Design review of the part built by this model. Coordinates are the model's own, in mm. A direction names the side the tool comes from. Round coordinates to 2 decimals unless told otherwise and drop trailing zeros. Loops run counter-clockwise (first coordinate to the right, second up) from the corner with the lowest first, then second, coordinate; pieces in that order, holes last. Notation, with made-up numbers: (40.25, 57.5) -> (86.25, 57.5) arc R17 cw to (86.25, 68.5) -> close; hole circle Ø8 at (36.5, 80.25). An arc over 180 degrees is marked (long way). Use a Markdown table: item, result. Add a question column.
from build123d import *

# Parameters (mm, degrees)
CYLINDER267_R                = 2
CYLINDER267_DEPTH            = 10
CYLINDER267_PITCH_ANGLE      = 90
BOX001027045199_W            = 3
BOX001027045199_H            = 8
BOX001027045199_DEPTH        = 8
FILLET045_R                  = 3
CUT239_PITCH_ANGLE           = 90
CYLINDER103_R                = 1.4
CYLINDER103_DEPTH            = 19
CYLINDER103_ROLL_ANGLE       = 90
CYLINDER105_R                = 1.4
CYLINDER105_DEPTH            = 19
CYLINDER105_ROLL_ANGLE       = 90
CYLINDER106_R                = 1.4
CYLINDER106_DEPTH            = 19
CYLINDER106_ROLL_ANGLE       = 90
CYLINDER027_R                = 1.4
CYLINDER027_DEPTH            = 19
CYLINDER027_ROLL_ANGLE       = 90
CYLINDER098_R                = 1
CYLINDER098_DEPTH            = 30
CYLINDER099_R                = 1
CYLINDER099_DEPTH            = 30
BOX001007_W                  = 4
BOX001007_H                  = 4.2
BOX001007_DEPTH              = 27
CYLINDER097_R                = 2.1
CYLINDER097_DEPTH            = 30
CYLINDER023_R                = 2.1
CYLINDER023_DEPTH            = 30
CYLINDER100_R                = 1
CYLINDER100_DEPTH            = 30
BOX001008_W                  = 4
BOX001008_H                  = 2
BOX001008_DEPTH              = 27
CYLINDER101_R                = 1
CYLINDER101_DEPTH            = 30
BOX001009_W                  = 4
BOX001009_H                  = 2
BOX001009_DEPTH              = 27
CYLINDER093_R                = 3.5
CYLINDER093_DEPTH            = 30
CYLINDER094_R                = 4.7
CYLINDER094_DEPTH            = 30
CYLINDER095_R                = 10
CYLINDER095_DEPTH            = 30
CYLINDER102_R                = 10
CYLINDER102_DEPTH            = 30
CYLINDER096_R                = 10
CYLINDER096_DEPTH            = 30
BOX001006_W                  = 39
BOX001006_H                  = 24
BOX001006_DEPTH              = 10
CHAMFER008_SIZE              = 1
CHAMFER014_SIZE              = 0.5
FUSION112154_ROLL_ANGLE      = 180
FUSION112154_PLACEMENT_ANGLE = -90


with BuildPart() as cylinder285:
    # Cylinder267 → Cylinder267 (new body)
    with BuildSketch(Plane.XY):
        Circle(CYLINDER267_R)
    extrude(amount=CYLINDER267_DEPTH)


with BuildPart() as cylinder285_1:
    # Cylinder267 pitch: moved
    add(cylinder285.part.rotate(Axis((0, 0, 0), (0, 1, 0)), CYLINDER267_PITCH_ANGLE))


with BuildPart() as cylinder285_2:
    # Cylinder267 placement: moved
    add(cylinder285_1.part.moved(Location((-3, 4, 4.5))))


with BuildPart() as cut239:
    # Box001027045199 → Box001027045199 (new body)
    with BuildSketch(Plane.XY):
        with Locations((1.5, 4)):
            Rectangle(BOX001027045199_W, BOX001027045199_H)
    extrude(amount=BOX001027045199_DEPTH)

    # Fillet045
    fillet045_edges = [cut239.edges().sort_by_distance(p)[0] for p in [
        (1.5, 0, 8),
        (1.5, 8, 8),
    ]]
    fillet(fillet045_edges, radius=FILLET045_R)

    # Cut239: cut Cylinder285
    add(cylinder285_2.part, mode=Mode.SUBTRACT)


with BuildPart() as cut239_1:
    # Cut239 pitch: moved
    add(cut239.part.rotate(Axis((0, 0, 0), (0, 1, 0)), CUT239_PITCH_ANGLE))


with BuildPart() as cut239_2:
    # Cut239 placement: moved
    add(cut239_1.part.moved(Location((25, -4, 10))))


with BuildPart() as cylinder103:
    # Cylinder103 → Cylinder103 (new body)
    with BuildSketch(Plane.XY):
        Circle(CYLINDER103_R)
    extrude(amount=CYLINDER103_DEPTH)


with BuildPart() as cylinder103_1:
    # Cylinder103 roll: moved
    add(cylinder103.part.rotate(Axis((0, 0, 0), (1, 0, 0)), CYLINDER103_ROLL_ANGLE))


with BuildPart() as cylinder103_2:
    # Cylinder103 placement: moved
    add(cylinder103_1.part.moved(Location((4, 24, 6))))


with BuildPart() as cylinder105:
    # Cylinder105 → Cylinder105 (new body)
    with BuildSketch(Plane.XY):
        Circle(CYLINDER105_R)
    extrude(amount=CYLINDER105_DEPTH)


with BuildPart() as cylinder105_1:
    # Cylinder105 roll: moved
    add(cylinder105.part.rotate(Axis((0, 0, 0), (1, 0, 0)), CYLINDER105_ROLL_ANGLE))


with BuildPart() as cylinder105_2:
    # Cylinder105 placement: moved
    add(cylinder105_1.part.moved(Location((-4, 24, 6))))


with BuildPart() as part_mirroring011:
    # Part__Mirroring011: instance of Cylinder105
    add(cylinder105_2.part.mirror(Plane(origin=(0, 0, 0), x_dir=(1, 0, 0), z_dir=(0, 1, 0))))


with BuildPart() as cylinder106:
    # Cylinder106 → Cylinder106 (new body)
    with BuildSketch(Plane.XY):
        Circle(CYLINDER106_R)
    extrude(amount=CYLINDER106_DEPTH)


with BuildPart() as cylinder106_1:
    # Cylinder106 roll: moved
    add(cylinder106.part.rotate(Axis((0, 0, 0), (1, 0, 0)), CYLINDER106_ROLL_ANGLE))


with BuildPart() as cylinder106_2:
    # Cylinder106 placement: moved
    add(cylinder106_1.part.moved(Location((4, 24, 6))))


with BuildPart() as part_mirroring012:
    # Part__Mirroring012: instance of Cylinder106
    add(cylinder106_2.part.mirror(Plane(origin=(0, 0, 0), x_dir=(1, 0, 0), z_dir=(0, 1, 0))))


with BuildPart() as m3_tap_a:
    # Cylinder027 → Cylinder027 (new body)
    with BuildSketch(Plane.XY):
        Circle(CYLINDER027_R)
    extrude(amount=CYLINDER027_DEPTH)


with BuildPart() as m3_tap_a_1:
    # Cylinder027 roll: moved
    add(m3_tap_a.part.rotate(Axis((0, 0, 0), (1, 0, 0)), CYLINDER027_ROLL_ANGLE))


with BuildPart() as m3_tap_a_2:
    # Cylinder027 placement: moved
    add(m3_tap_a_1.part.moved(Location((-4, 24, 6))))

    # Fusion062: union Cylinder103, Part__Mirroring011, Part__Mirroring012
    add(cylinder103_2.part)
    add(part_mirroring011.part)
    add(part_mirroring012.part)


with BuildPart() as cylinder109:
    # Cylinder098 → Cylinder098 (new body)
    with BuildSketch(Plane(origin=(17, -4.5, -12.5), x_dir=(1, 0, 0), z_dir=(0, 0, 1))):
        Circle(CYLINDER098_R)
    extrude(amount=CYLINDER098_DEPTH)


with BuildPart() as cylinder110:
    # Cylinder099 → Cylinder099 (new body)
    with BuildSketch(Plane(origin=(17, 4.5, -12.5), x_dir=(1, 0, 0), z_dir=(0, 0, 1))):
        Circle(CYLINDER099_R)
    extrude(amount=CYLINDER099_DEPTH)


with BuildPart() as cube046:
    # Box001007 → Box001007 (new body)
    with BuildSketch(Plane(origin=(13, -2.1, -11), x_dir=(1, 0, 0), z_dir=(0, 0, 1))):
        with Locations((2, 2.1)):
            Rectangle(BOX001007_W, BOX001007_H)
    extrude(amount=BOX001007_DEPTH)


with BuildPart() as cylinder108:
    # Cylinder097 → Cylinder097 (new body)
    with BuildSketch(Plane(origin=(17, 0, -12.5), x_dir=(1, 0, 0), z_dir=(0, 0, 1))):
        Circle(CYLINDER097_R)
    extrude(amount=CYLINDER097_DEPTH)


with BuildPart() as cylinder111:
    # Cylinder023 → Cylinder023 (new body)
    with BuildSketch(Plane(origin=(13, 0, -12.5), x_dir=(1, 0, 0), z_dir=(0, 0, 1))):
        Circle(CYLINDER023_R)
    extrude(amount=CYLINDER023_DEPTH)


with BuildPart() as cylinder112:
    # Cylinder100 → Cylinder100 (new body)
    with BuildSketch(Plane(origin=(13, -4.5, -12.5), x_dir=(1, 0, 0), z_dir=(0, 0, 1))):
        Circle(CYLINDER100_R)
    extrude(amount=CYLINDER100_DEPTH)


with BuildPart() as cube047:
    # Box001008 → Box001008 (new body)
    with BuildSketch(Plane(origin=(13, -5.5, -11), x_dir=(1, 0, 0), z_dir=(0, 0, 1))):
        with Locations((2, 1)):
            Rectangle(BOX001008_W, BOX001008_H)
    extrude(amount=BOX001008_DEPTH)


with BuildPart() as cylinder113:
    # Cylinder101 → Cylinder101 (new body)
    with BuildSketch(Plane(origin=(13, 4.5, -12.5), x_dir=(1, 0, 0), z_dir=(0, 0, 1))):
        Circle(CYLINDER101_R)
    extrude(amount=CYLINDER101_DEPTH)


with BuildPart() as motor_slots:
    # Box001009 → Box001009 (new body)
    with BuildSketch(Plane(origin=(13, 3.5, -11), x_dir=(1, 0, 0), z_dir=(0, 0, 1))):
        with Locations((2, 1)):
            Rectangle(BOX001009_W, BOX001009_H)
    extrude(amount=BOX001009_DEPTH)

    # Fusion058: union Cylinder109, Cylinder110, Cube046, Cylinder108, Cylinder111, Cylinder112, Cube047, Cylinder113
    add(cylinder109.part)
    add(cylinder110.part)
    add(cube046.part)
    add(cylinder108.part)
    add(cylinder111.part)
    add(cylinder112.part)
    add(cube047.part)
    add(cylinder113.part)


with BuildPart() as cylinder104:
    # Cylinder093 → Cylinder093 (new body)
    with BuildSketch(Plane.XY.offset(-12)):
        Circle(CYLINDER093_R)
    extrude(amount=CYLINDER093_DEPTH)


with BuildPart() as cylinder094:
    # Cylinder094 → Cylinder094 (new body)
    with BuildSketch(Plane.XY.offset(-21.5)):
        Circle(CYLINDER094_R)
    extrude(amount=CYLINDER094_DEPTH)


with BuildPart() as cylinder095:
    # Cylinder095 → Cylinder095 (new body)
    with BuildSketch(Plane.XY.offset(-25.5)):
        Circle(CYLINDER095_R)
    extrude(amount=CYLINDER095_DEPTH)


with BuildPart() as cylinder114:
    # Cylinder102 → Cylinder102 (new body)
    with BuildSketch(Plane(origin=(15, 0, -25.5), x_dir=(1, 0, 0), z_dir=(0, 0, 1))):
        Circle(CYLINDER102_R)
    extrude(amount=CYLINDER102_DEPTH)


with BuildPart() as fusion060:
    # Cylinder096 → Cylinder096 (new body)
    with BuildSketch(Plane(origin=(16, 0, -25.5), x_dir=(1, 0, 0), z_dir=(0, 0, 1))):
        Circle(CYLINDER096_R)
    extrude(amount=CYLINDER096_DEPTH)

    # Fusion059: union Cylinder104, Cylinder094, Cylinder095, Cylinder114
    add(cylinder104.part)
    add(cylinder094.part)
    add(cylinder095.part)
    add(cylinder114.part)

    # Fusion060: union motor-slots
    add(motor_slots.part)


with BuildPart() as gearbox001:
    # Box001006 → Box001006 (new body)
    with BuildSketch(Plane(origin=(-12, -12, 0), x_dir=(1, 0, 0), z_dir=(0, 0, 1))):
        with Locations((19.5, 12)):
            Rectangle(BOX001006_W, BOX001006_H)
    extrude(amount=BOX001006_DEPTH)

    # Cut005: cut Fusion060
    add(fusion060.part, mode=Mode.SUBTRACT)

    # Chamfer008
    chamfer008_edges = [gearbox001.edges().sort_by_distance(p)[0] for p in [
        (12, 4.5, 4.5),
        (15, 3.5, 4.5),
        (17.707107, 3.792893, 4.5),
        (17.707107, 5.207107, 4.5),
        (15, 5.5, 4.5),
        (17.707107, -5.207107, 4.5),
        (17.707107, -3.792893, 4.5),
        (15, -3.5, 4.5),
        (12, -4.5, 4.5),
        (15, -5.5, 4.5),
    ]]
    chamfer(chamfer008_edges, length=CHAMFER008_SIZE)

    # Cut045: cut M3-tap-a
    add(m3_tap_a_2.part, mode=Mode.SUBTRACT)

    # Chamfer014
    chamfer014_edges = [gearbox001.edges().sort_by_distance(p)[0] for p in [
        (18.484924, 1.484924, 10),
        (15, 2.1, 10),
        (10.9, 0, 10),
        (15, -2.1, 10),
        (18.484924, -1.484924, 10),
    ]]
    chamfer(chamfer014_edges, length=CHAMFER014_SIZE)

    # Fusion112154: union Cut239
    add(cut239_2.part)


with BuildPart() as gearbox001_1:
    # Fusion112154 roll: moved
    add(gearbox001.part.rotate(Axis((0, 0, 0), (1, 0, 0)), FUSION112154_ROLL_ANGLE))


with BuildPart() as gearbox001_2:
    # Fusion112154 placement: moved
    add(gearbox001_1.part.moved(Location((61.5, 15, 17.5))).rotate(Axis((61.5, 15, 17.5), (0, 0, 1)), FUSION112154_PLACEMENT_ANGLE))


solid = gearbox001_2.part
1. For faces 1 (the face through (61.549, 4.235, 7.865)), 2 (the face through (52.95, 12.4, 11.44)), 3 (the face through (63.6, 0, 11)), 4 (the face through (67.5, 0, 12.5)), 5 (the face through (57.5, -13, 9)), list the 3-axis set-ups (+Z, -Z, +X, -X, +Y, -Y) from which the entire face can be reached by the end or side of a thin tool; tool diameter is ignored.
2. To check wall thickness, follow probe 1 along Y at (x, z) = (54.25, 11.5); probe 2 along X at (y, z) = (0.5, 10); probe 3 along X at (y, z) = (15, 8.3). State the ranges of each line that lie inside material, in increasing order. Write a range as from..to.
3. Insertion check: P1, Ø0.9, axis at y = -13.5, z = 8.5, coming from the -X side; P2, Ø2, axis at y = 19, z = 11.5, coming from the -X side; P3, Ø5, axis at x = 53, z = 11.5, coming from the -Y side. Each pin has a flat end and moves straight along its axis. Give the tip position at first contact, or say it passes through.
4. Consider section A-A on x = 61.5. State the section outline as (y, z) points, plus the area to 3 significant figures.
5. Mouldability with a two-part tool opening along Y and no side actions: class faces 6 (the face through (67, 0, 10)), 7 (the face through (61, -18, 9)), 8 (the face through (61, 5, 7.5)) as +Y half, -Y half, draft (parallel to the pull), parting line (faces both ways), or undercut.
6. Consider section C-C on y = -1. State the section outline as (x, z) points.
7. Consider section D-D on x = 52.75. State the section outline as (y, z) points, plus the area to 3 significant figures.
8. Consider section B-B on y = 15. State the section outline as (x, z) points, plus the area to 3 significant figures.
Verdict:
| question | item | result |
|---|---|---|
| 1 | face 1 | -Z |
| 1 | face 2 | -X |
| 1 | face 3 | +Z, -Z |
| 1 | face 4 | +Z |
| 1 | face 5 | +Z, -Z, -X, -Y |
| 2 | probe 1 | y = -12..9.6, 12.4..17.6, 20.4..27 |
| 2 | probe 2 | x = 49.5..56, 58..59.4, 63.6..65, 67..73.5 |
| 2 | probe 3 | x = 49.5..58, 65..73.5 |
| 3 | P1 | stops at x = 57.5 |
| 3 | P2 | stops at x = 56.5 |
| 3 | P3 | stops at y = -12 |
| 4 | outline | (-18, 7.5) -> (-16.5, 7.5) -> (-16.5, 10.5) -> (-18, 10.5) -> close; (-12.5, 7.5) -> (-4.6, 7.5) -> (-4.1, 8) -> (-4.1, 13) -> (-11, 13) -> (-11, 17.5) -> (-12, 17.5) -> (-12, 10.5) -> (-12.5, 10.5) -> close; (4.1, 8) -> (4.6, 7.5) -> (11.5, 7.5) -> (11.5, 9) -> (10.3, 9) -> (10.3, 13) -> (4.1, 13) -> close; (18.5, 7.5) -> (27, 7.5) -> (27, 17.5) -> (25, 17.5) -> (25, 13) -> (19.7, 13) -> (19.7, 9) -> (18.5, 9) -> close |
| 4 | area | 141 mm² |
| 5 | face 6 | undercut |
| 5 | face 7 | -Y half |
| 5 | face 8 | draft |
| 6 | outline | (49.5, 7.5) -> (56, 7.5) -> (56, 12) -> (55, 13) -> (51.5, 13) -> (51.5, 17.5) -> (49.5, 17.5) -> close; (58, 7.5) -> (58.9, 7.5) -> (59.4, 8) -> (59.4, 13) -> (59, 13) -> (58, 12) -> close; (63.6, 8) -> (64.1, 7.5) -> (65, 7.5) -> (65, 12) -> (64, 13) -> (63.6, 13) -> close; (67, 7.5) -> (73.5, 7.5) -> (73.5, 17.5) -> (71.5, 17.5) -> (71.5, 13) -> (68, 13) -> (67, 12) -> close |
| 7 | outline | (-12, 7.5) -> (27, 7.5) -> (27, 17.5) -> (19.84, 17.5) -> (19.84, 13) -> (10.16, 13) -> (10.16, 17.5) -> (4.84, 17.5) -> (4.84, 13) -> (-5.84, 13) -> (-5.84, 17.5) -> (-12, 17.5) -> close; hole circle Ø2.8 at (11, 11.5); hole circle Ø2.8 at (19, 11.5) |
| 7 | area | 286 mm² |
| 8 | outline | (49.5, 7.5) -> (58, 7.5) -> (58, 9) -> (56.8, 9) -> (56.8, 13) -> (51.5, 13) -> (51.5, 17.5) -> (49.5, 17.5) -> close; (65, 7.5) -> (73.5, 7.5) -> (73.5, 17.5) -> (71.5, 17.5) -> (71.5, 13) -> (66.2, 13) -> (66.2, 9) -> (65, 9) -> close |
| 8 | area | 102 mm² |
